Design review of the part shown in the three views and the two pictorial views. Dimensions are in mm from the part's minimum x, y and z. A direction names the side the tool comes from. Coordinates: 2 decimals unless noted, no trailing zeros. Write each loop counter-clockwise with the first axis right and the second up, starting at its lowest first coordinate (ties: lowest second). Pieces come first, ordered by that corner, then holes. Notation, with made-up numbers: M 35,35.5 L 46,35.5 A36 ccw 46,69.5 Z; hole C 67,1 d6. An arc over 180 degrees is marked long. Answer as a JSON object with one key per item and string values.
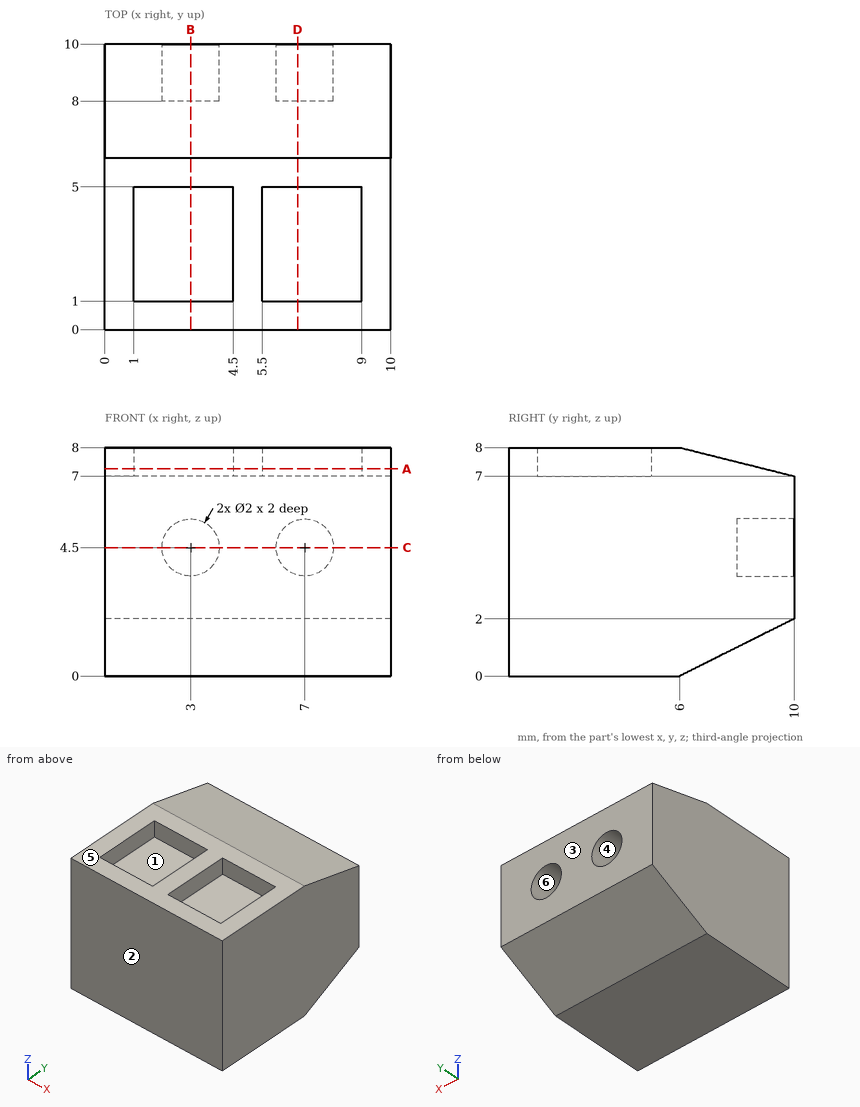
(1) Wall thickness on line 1 along X through (y, z) = (9.25, 4.5); line 2 along X through (y, z) = (9.25, 3.75); line 3 along Y through (x, z) = (3.75, 1.5): over which ranges is each line inside the solid? List them lowest first. Write a range as from..to.
Results list:
{"line 1": "0..2, 4..6, 8..10", "line 2": "0..2.34, 3.66..6.34, 7.66..10", "line 3": "0..9"}
(2) Add section D-D on x = 6.75. Give the boundary of the cut face in (y, z), and give its area (3 significant figures).
Results list:
{"outline": "M 0,0 L 6,0 L 10,2 L 10,3.53 L 8,3.53 L 8,5.47 L 10,5.47 L 10,7 L 6,8 L 5,8 L 5,7 L 1,7 L 1,8 L 0,8 Z", "area": "66.1 mm²"}
(3) Draft analysis for pull direction Z (two halves, no side actions). For the marked faces 3, 4, 5 and 6, state which applies: released by +Z, released by -Z, zero draft, split by the parting line, or undercut.
Results list:
{"face 3": "zero draft", "face 4": "undercut", "face 5": "released by +Z", "face 6": "undercut"}
(4) Add section C-C on z = 4.5. Give the boundary of the cut face in (x, y), and give its area (3 significant figures).
Results list:
{"outline": "M 0,0 L 10,0 L 10,10 L 8,10 L 8,8 L 6,8 L 6,10 L 4,10 L 4,8 L 2,8 L 2,10 L 0,10 Z", "area": "92.0 mm²"}
(5) For the marked faces 1 and 2, list the 3-axis set-ups (+Z, -Z, +X, -X, +Y, -Y) from which the entire face can be reached by the end or side of a thin tool; tool diameter is ignored.
Results list:
{"face 1": "+Z", "face 2": "+Z, -Z, +X, -X, -Y"}
(6) Add section A-A on z = 7.25. Give the boundary of the cut face in (x, y), and give its area (3 significant figures).
Results list:
{"outline": "M 0,0 L 10,0 L 10,9 L 0,9 Z; hole M 1,1 L 4.5,1 L 4.5,5 L 1,5 Z; hole M 5.5,1 L 9,1 L 9,5 L 5.5,5 Z", "area": "62.0 mm²"}
(7) Add section B-B on x = 3. Give the boundary of the cut face in (y, z), and give its area (3 significant figures).
Results list:
{"outline": "M 0,0 L 6,0 L 10,2 L 10,3.5 L 8,3.5 L 8,5.5 L 10,5.5 L 10,7 L 6,8 L 5,8 L 5,7 L 1,7 L 1,8 L 0,8 Z", "area": "66.0 mm²"}
(8) For pin 1 Ø1.1 at (x, z) = (6.5, 7.5) entering from +Y, flat-tipped, find the tip position at first contact; note if it passes through.
Results list:
{"pin 1": "y = 10"}
